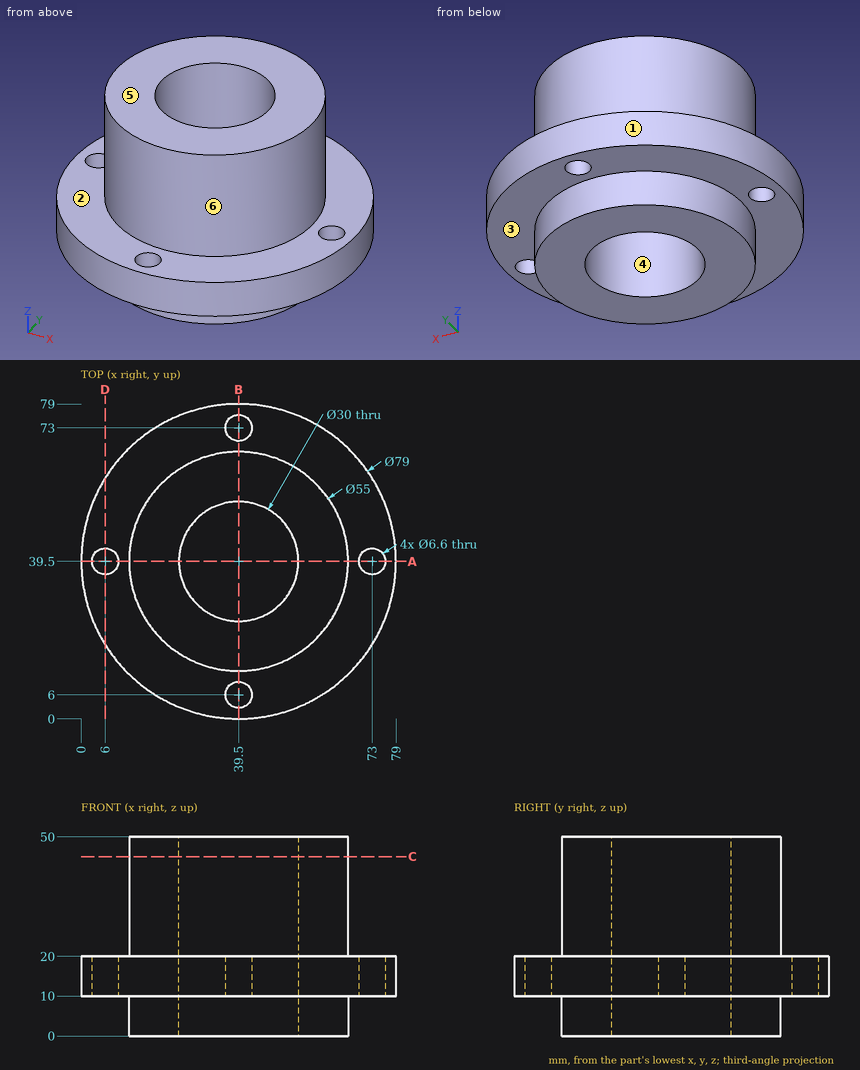
Answer from the drawing. Dimensions are ordinates in mm from the lowest x, y and z of the part. A direction names the side the tool comes from. Give positions to 0.01 mm unless a question says otherwise; leave off trailing zeros. Write each loop counter-clockwise with the first axis right and the second up, starting at its lowest first coordinate (ties: lowest second). Pieces come first, ordered by that corner, then holes. Notation, with made-up numbers: (72.25, 6) - (85.25, 6) arc R21 ccw to (85.25, 34) - close; hole circle Ø4 at (21, -13). An arc over 180 degrees is marked (long way). Answer in a Markdown table with one row per item. Add a question column.
Item 1: Section C-C, the plane z = 45 is taken. Write down the section's boundary in (x, y), and give its area (3 significant figures).
Item 2: Find the intervals of material crossed by L1, parallel to Y at x = 39.5, z = 27; L2, parallel to X at y = 42, z = 15.5; L3, parallel to Y at x = 39, z = 12, in increasing order.
Item 3: Section A-A, the plane y = 39.5 is taken. Write down the section's boundary in (x, z).
Item 4: A tool of negligible diameter and unlimited length cuts with its end or side. For the marked faces 1, 2 and 3, from which of +Z, -Z, +X, -X, +Y, -Y can it reach the whole face along a straight path? Write none if from no direction.
Item 5: Section D-D, the plane x = 6 is taken. Write down the section's boundary in (y, z).
Item 6: Flat-ended cylindrical pins translate along their axes: P1, Ø12, axis at x = 39.5, z = 18.5, coming from the -Y side; P2, Ø7.5, axis at x = 39.5, y = 73, coming from the -Z side; P3, Ø6, axis at y = 64, z = 37, coming from the +X side; P4, Ø5.5, axis at x = 39.5, y = 6, coming from the +Z side. Find the tip coordinate at first contact, or state that the pin passes through.
Item 7: Determine the mould class of the marked faces 4, 5 and 6 for opening direction X: pulls with the +X half, pulls with the -X half, needs draft (parallel to the pull), parting line crosses it, or undercut.
Recorded:
| question | item | result |
|---|---|---|
| 1 | outline | circle Ø55 at (39.5, 39.5); hole circle Ø30 at (39.5, 39.5) |
| 1 | area | 1,670 mm2 |
| 2 | L1 | y = 12 to 24.5, 54.5 to 67 |
| 2 | L2 | x = 0.08 to 3.85, 8.15 to 24.71, 54.29 to 70.85, 75.15 to 78.92 |
| 2 | L3 | y = 0 to 2.74, 9.26 to 24.51, 54.49 to 69.74, 76.26 to 79 |
| 3 | outline | (0, 10) - (2.7, 10) - (2.7, 20) - (0, 20) - close; (9.3, 10) - (12, 10) - (12, 0) - (24.5, 0) - (24.5, 50) - (12, 50) - (12, 20) - (9.3, 20) - close; (54.5, 0) - (67, 0) - (67, 10) - (69.7, 10) - (69.7, 20) - (67, 20) - (67, 50) - (54.5, 50) - close; (76.3, 10) - (79, 10) - (79, 20) - (76.3, 20) - close |
| 4 | face 1 | +Z, -Z |
| 4 | face 2 | +Z |
| 4 | face 3 | -Z |
| 5 | outline | (18.57, 10) - (36.2, 10) - (36.2, 20) - (18.57, 20) - close; (42.8, 10) - (60.43, 10) - (60.43, 20) - (42.8, 20) - close |
| 6 | P1 | stops at y = 0 |
| 6 | P2 | stops at z = 10 |
| 6 | P3 | stops at x = 56.65 |
| 6 | P4 | passes through |
| 7 | face 4 | undercut |
| 7 | face 5 | needs draft |
| 7 | face 6 | parting line crosses it |
